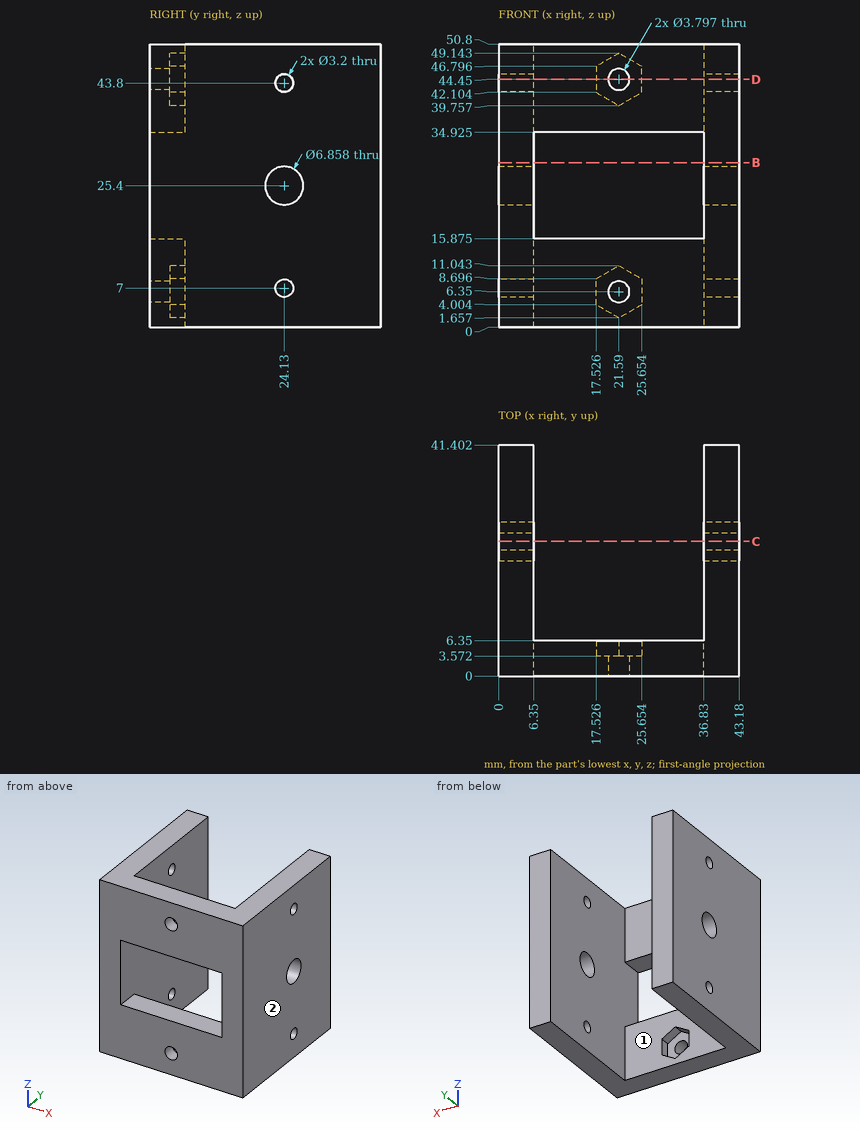
Verification items for this drawing (mm, ordinates from the low corner). A direction names the side the tool comes from. Give positions to 0.01 mm unless a question says otherwise; leave off trailing zeros. Write each loop counter-clockwise with the first axis right and the second up, starting at its lowest first coordinate (ties: lowest second). Pieces come first, ordered by that corner, then holes. Notation, with made-up numbers: (-18, 22) -> (16, 22) arc R37 ccw to (16, 60) -> close; hole circle Ø5 at (5.5, 31.25). An arc over 180 degrees is marked (long way). Use one line per item in the form item = value.
Item 1: Scan lines: line 1 (Z direction, x = 39.25, y = 24.13); line 2 (Z direction, x = 21.59, y = 2.1) (1 decimal); line 3 (X direction, y = 32.5, z = 28). Record each from-to range of solid material in increasing order.
Results list:
line_1 = 0 to 5.4, 8.6 to 21.97, 28.83 to 42.2, 45.4 to 50.8
line_2 = 0 to 4.5, 8.2 to 15.9, 34.9 to 42.6, 46.3 to 50.8
line_3 = 0 to 6.35, 36.83 to 43.18
Item 2: Sectioned sample at D-D on z = 44.45. Enter the section's corners in (x, y).
Results list:
outline = (0, 0) -> (19.69, 0) -> (19.69, 3.57) -> (17.53, 3.57) -> (17.53, 6.35) -> (6.35, 6.35) -> (6.35, 22.67) -> (0, 22.67) -> close; (0, 25.59) -> (6.35, 25.59) -> (6.35, 41.4) -> (0, 41.4) -> close; (23.49, 0) -> (43.18, 0) -> (43.18, 22.67) -> (36.83, 22.67) -> (36.83, 6.35) -> (25.65, 6.35) -> (25.65, 3.57) -> (23.49, 3.57) -> close; (36.83, 25.59) -> (43.18, 25.59) -> (43.18, 41.4) -> (36.83, 41.4) -> close
Item 3: Access from +Z, -Z, +X, -X, +Y, -Y to the whole of each face (thin tool, end or side, straight path). Record for the marked faces 1 and 2.
Results list:
face_1 = +Z, -Z, +Y
face_2 = +Z, -Z, +X, +Y, -Y
Item 4: Sectioned sample at C-C on y = 24.13. Count the separate pieces of the cut face and the enclosed holes in it, plus the area to 3 significant figures.
Results list:
separate_pieces = 8
enclosed_holes = 0
area = 477 mm2
Item 5: Sectioned sample at B-B on z = 29.5. Enter the section's corners in (x, y), plus the area to 3 significant figures.
Results list:
outline = (0, 0) -> (6.35, 0) -> (6.35, 41.4) -> (0, 41.4) -> close; (36.83, 0) -> (43.18, 0) -> (43.18, 41.4) -> (36.83, 41.4) -> close
area = 526 mm2
Item 6: Depth check by flat-ended pin: pin 1 Ø3.5 at (y, z) = (24.13, 7) entering from +X; pin 2 Ø8 at (x, z) = (17, 4.5) entering from +Y; pin 3 Ø6 at (x, z) = (21.59, 6.35) entering from +Y. Enter the tip coordinate at first touch or a pass-through.
Results list:
pin_1 = 43.18
pin_2 = 6.35
pin_3 = 3.57
